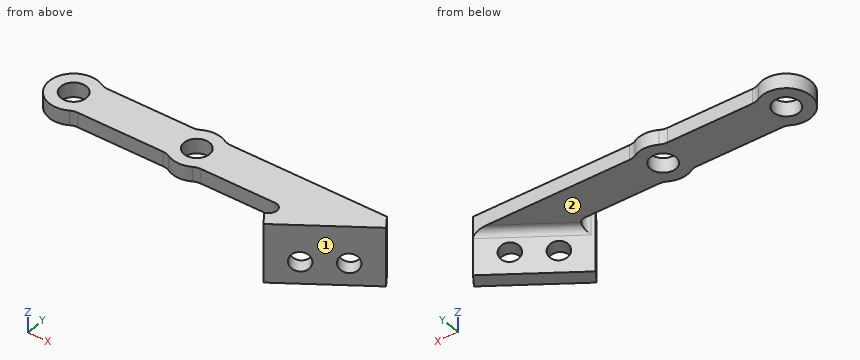
Autodesk Inventor part; units mm, degrees
ref_plane "YZ Plane" through (0, 0, 0) normal (1, 0, 0) x (0, 1, 0)
ref_plane "XZ Plane" through (0, 0, 0) normal (0, 1, 0) x (-1, 0, 0)
ref_plane "XY Plane" through (0, 0, 0) normal (0, 0, 1) x (1, 0, 0)
sketch "スケッチ1" plane through (0, 0, 0) normal (0, 0, 1) x (1, 0, 0)
  line L0 (0, 0) -> (45, 0) construction
  line L1 (0, -4) -> (45, -4)
  line L2 (45, 4) -> (0, 4)
  arc A0 (0, 4) -> (0, -4) centre (0, 0) ccw
  arc A1 (45, -4) -> (45, 4) centre (45, 0) ccw
  circle A2 centre (0, 0) radius 2.6
  circle A3 centre (25.1, 0) radius 2.6
  line L3 (36.8368, 4) -> (49, 4)
  line L4 (49, 4) -> (49, -4)
  line L5 (49, -4) -> (36.8368, -4)
  line L6 (36.8368, -4) -> (36.8368, 4)
  circle A4 centre (0, 0) radius 5
  circle A5 centre (25.1, 0) radius 5
  point P0 (22.5, 0)
  dimension "d0" = 4
  dimension "d1" = 45
  dimension "d2" = 5.2
  dimension "d3" = 5.2
  dimension "d4" = 25.1
  dimension "d7" = 12.1632
  dimension "d8" = 8
  dimension "d9" = 4
  dimension "d34" = 10
  dimension "d35" = 10
extrude "押し出し1" add sketch "スケッチ1" along normal blind 3
draft "面の勾配1" angle 56 pull direction (0, -1, 0) faces at (49, -1.3333, 1) fixed edges at (49, -4, 1.5)
ref_plane "作業平面1" through (60.8605, 4, 0) normal (0.5591929, -0.8290376, 0) x (0.8290376, 0.5591929, 0)
sketch "スケッチ3" plane through (60.8605, 4, 0) normal (0.5591929, -0.8290376, 0) x (0.8290376, 0.5591929, 0)
  line L0 (0, -9) -> (-20, -9)
  line L1 (-20, -9) -> (-20, 3)
  line L2 (-20, 3) -> (0, 3)
  line L3 (0, 3) -> (0, -9)
  line L4 (0, 0) -> (0, 3)
  circle A0 centre (-14, -4.5) radius 2
  circle A1 centre (-6, -4.5) radius 2
  line L5 (-31.6332, 3) -> (-14.3063, 3)
  point P0 (-52.6924, 0)
  point P1 (2.1488, 1.5)
  dimension "d12" = 20
  dimension "d13" = 0
  dimension "d14" = 12
  dimension "d15" = 1.5
  dimension "d21" = 4
  dimension "d22" = 4
  dimension "d25" = 6
  dimension "d26" = 6
  dimension "d29" = 6
  dimension "d30" = 6
  dimension "d39" = 0
extrude "押し出し3" add sketch "スケッチ3" along normal blind 3
fillet "フィレット2" radius 3 6 edges at (3, 4, 1.5) (28.1, 4, 1.5) (22.1, 4, 1.5) (3, -4, 1.5) (28.1, -4, 1.5) (22.1, -4, 1.5)
fillet "フィレット5" radius 1.5 2 edges at (54.9302, 0, 0) (49, -4, 1.5)
equation "\"d3\" = d2"
equation "\"d21\" = d19"
equation "\"d22\" = d19"
equation "\"d29\" = d28"
equation "\"d30\" = d24"
equation "\"d28\" = d24"
properties part number "leg"
Read the model definition and answer for the solid it produces. Units are mm, in the model's axes. Face numbers are marked on the shaded views. A direction names the side the tool comes from. Coordinates: 2 decimals unless noted, no trailing zeros. Order: outer loops, then holes, each group sorted by start corner. A loop starts at its lowest first (then second) coordinate and runs counter-clockwise, first axis right, second up. Notation, with made-up numbers: (33, 35.25) -> (41, 35.25) arc R29 cw to (41, 63.25) -> close; hole circle Ø7 at (36, -33.75). An arc over 180 degrees is marked (long way). Answer as a JSON object with one key per item and string values.
1) A cutting plane is placed at D-D, the plane x = 10. Determine the outline of the cut face in (y, z), plus the area to 3 significant figures.
Model answer:
{"outline": "(-4, 0) -> (4, 0) -> (4, 3) -> (-4, 3) -> close", "area": "24.0 mm²"}
2) Each of these flat-tipped pins is pushed along its axis until it touches: pin 1 (1.5 mm diameter, centred on x = 11, z = 1, fed in from +Y); pin 2 (5 mm diameter, centred on x = 41, y = 1, fed in from -Z); pin 3 (4 mm diameter, centred on x = 25.1, y = 0, fed in from +Z); pin 4 (5 mm diameter, centred on y = -4, z = 1.5, fed in from +X). Where does it stop, or does it pass through?
Model answer:
{"pin 1": "stops at y = 4", "pin 2": "stops at z = 0", "pin 3": "passes through", "pin 4": "stops at x = 58.07"}
3) Consider line 1 along Y through (x, z) = (25.1, 2.35); line 2 along Z through (x, y) = (27, -4.25); line 3 along X through (y, z) = (2, 0.75). Determine where each line is inside the solid, lowest interval first. Write a range as from..to.
Model answer:
{"line 1": "y = -5..-2.6, 2.6..5", "line 2": "z = 0..3", "line 3": "x = -4.58..-1.66, 1.66..23.44, 26.76..62.21"}
4) A cutting plane is placed at C-C, the plane z = 1.25. Determine the outline of the cut face in (x, y) (1 decimal), plus the area to 3 significant figures.
Model answer:
{"outline": "(2.4, -4.4) arc R3 cw to (3.9, -4) -> (21.2, -4) arc R3 cw to (22.7, -4.4) arc R5 ccw to (27.5, -4.4) arc R3 cw to (29, -4) -> (44.1, -4) arc R1.5 cw to (44.9, -6.7) -> (44.3, -7.2) -> (46, -9.7) -> (62.5, 1.5) -> (60.9, 4) -> (29, 4) arc R3 cw to (27.5, 4.4) arc R5 ccw to (22.7, 4.4) arc R3 cw to (21.2, 4) -> (3.9, 4) arc R3 cw to (2.4, 4.4) arc R5 ccw (long way) to start; hole circle Ø5.2 at (0, 0); hole circle Ø5.2 at (25.1, 0)", "area": "513 mm²"}
5) A cutting plane is placed at B-B, the plane z = -3.25. Determine the outline of the cut face in (x, y).
Model answer:
{"outline": "(44.28, -7.18) -> (45.96, -9.67) -> (49.64, -7.19) -> (47.96, -4.7) -> close; (50.55, -2.96) -> (52.23, -5.44) -> (56.27, -2.72) -> (54.59, -0.23) -> close; (57.18, 1.52) -> (58.86, -0.97) -> (62.54, 1.51) -> (60.86, 4) -> close"}
6) A cutting plane is placed at A-A, the plane x = 25.1. Determine the outline of the cut face in (y, z), plus the area to 3 significant figures.
Model answer:
{"outline": "(-5, 0) -> (-2.6, 0) -> (-2.6, 3) -> (-5, 3) -> close; (2.6, 0) -> (5, 0) -> (5, 3) -> (2.6, 3) -> close", "area": "14.4 mm²"}
7) A tool of negligible diameter and unlimited length cuts with its end or side. For the marked faces 1 and 2, from which of +Z, -Z, +X, -X, +Y, -Y can it reach the whole face along a straight path? Write none if from no direction.
Model answer:
{"face 1": "+Z, -Z, +X, -Y", "face 2": "-Z, -X, +Y"}
